Geometry check sheet. Reference: the model listing, model coordinates, mm. A direction names the side the tool comes from. Give positions to 0.01 mm unless a question says otherwise; leave off trailing zeros. Loops run counter-clockwise (first coordinate to the right, second up) from the corner with the lowest first, then second, coordinate; pieces in that order, holes last.
1. Cross-section at A-A, the plane y = 12.5. Record the cut outline in (x, z).
2. Cross-section at B-B, the plane z = -22.25. Record the cut outline in (x, y).
3. Release check for a two-part mould opening along X. For faces 1 (the flat face through (-29.572, 12.3, -31.3)), 2 (the flat face through (-14.5, 25, -38.8)), 3 (the cylindrical face through (-2.767, 22.487, -38.843)) record: +X half, -X half, draft (parallel to the pull), parting line (faces both ways), or undercut.
4. Tool access check on faces 4 (the cylindrical face through (-21.14, 4.45, -38.84)), 5 (the flat face through (-29.072, 12.3, -31.3)). Record the directions out of +Z, -Z, +X, -X, +Y, -Y that give a thin tool (end or side, any length) a straight path to the whole face; none if there is none.
5. Cross-section at D-D, the plane x = -2.5. Record the cut outline in (y, z).
6. Material ranges on L1, parallel to Z at x = -22.5, y = 1.5; L2, parallel to X at y = 24, z = -26.25, recorded low to high.
7. Cross-section at C-C, the plane y = 4. Record the cut outline in (x, z), plus the area to 3 significant figures.
8. Go/stop test with flat-tipped pins: pin 1 Ø7.5 at (x, y) = (-10, 14) entering from +Z; pin 2 Ø12.5 at (y, z) = (10.5, -24) entering from +X. Record where each tip stops, or that it passes through.
Autodesk Inventor part; units mm, degrees
ref_plane "YZ Plane" through (0, 0, 0) normal (1, 0, 0) x (0, 1, 0)
ref_plane "XZ Plane" through (0, 0, 0) normal (0, 1, 0) x (-1, 0, 0)
ref_plane "XY Plane" through (0, 0, 0) normal (0, 0, 1) x (1, 0, 0)
sketch "草圖1" plane through (0, 0, 0) normal (0, 1, 0) x (-1, 0, 0)
  line L0 (29.5719, -39.0966) -> (29.5719, -13.0966)
  line L1 (29.5719, -39.0966) -> (-0.4281, -39.0966)
  point P0 (0, 0)
  dimension "d0" = 26
  dimension "d2" = 90
  dimension "d3" = 30
contour flange "輪廓線凸緣1" sketch "草圖1" thickness 0.5 bend radius 0.5 width 25 along (0, 1, 0) mid plane no both sides no wall seen from (-29.5719, 0, -26.0966) lies toward (1, 0, 0) curves L0 L1
bend "折彎1"
corner "轉角1"
sketch "草圖2" plane through (-29.0719, 0, -13.0966) normal (1, 0, 0) x (0, 0, -1)
  circle A0 centre (12.5, 12.5) radius 12.5
  line L0 (0, 25) -> (25, 25)
  line L1 (0, 0) -> (0, 25)
  line L2 (0, 0) -> (25, 0)
  point P0 (-13.0966, 0)
  point P1 (0, 12.5)
  point P2 (12.5, 25)
  point P3 (12.5, 0)
  dimension "d15" = 25
extrude "擠出1" cut sketch "草圖2" against normal up to surface (0.5 mm away) contours A0 L1 L0 | L2 L1 A0
sketch "草圖3" plane through (-29.0719, 0, -38.0966) normal (1, 0, 0) x (0, 0, -1)
  arc A0 (-12.5, 25) -> (-12.5, 0) centre (-12.5, 12.5) ccw
  circle A1 centre (-12.5, 21) radius 1.5
  circle A2 centre (-12.5, 4) radius 1.5
  point P0 (-38.0966, 0)
  dimension "d18" = 3
  dimension "d19" = 17
  dimension "d20" = 8.5
  dimension "d21" = 3
extrude "擠出2" cut sketch "草圖3" against normal up to surface (0.5 mm away)
sketch "草圖4" plane through (0.4281, 0, -38.5966) normal (0, 0, 1) x (1, 0, 0)
  circle A0 centre (-23, 21) radius 1.5
  circle A1 centre (-3, 21) radius 1.5
  circle A2 centre (-23, 4) radius 1.5
  circle A3 centre (-3, 4) radius 1.5
  line L0 (0, 0) -> (0, 25)
  line L1 (-3, 21) -> (-3, 4)
  line L2 (-3, 12.5) -> (-13.1347, 12.5)
  line L3 (-29, 25) -> (0, 25)
  point P0 (-0.4281, 0)
  dimension "d24" = 20
  dimension "d25" = 3
  dimension "d26" = 3
  dimension "d27" = 3
  dimension "d28" = 3
  dimension "d29" = 17
  dimension "d30" = 3
  dimension "d31" = 12.5
extrude "擠出3" cut sketch "草圖4" against normal up to surface (0.5 mm away)
sketch "草圖5" plane through (-29.0719, 0, -38.0966) normal (1, 0, 0) x (0, 0, -1)
  arc A0 (-12.5, 25) -> (-12.5, 0) centre (-12.5, 12.5) ccw
  circle A1 centre (-12.5, 12.5) radius 5.5
  point P0 (-38.0966, 0)
  dimension "d34" = 11
extrude "擠出4" cut sketch "草圖5" against normal up to surface (0.5 mm away)
equation "\"d4\" = 厚度"
equation "\"d5\" = 折彎離隙寬度"
equation "\"d6\" = 折彎離隙深度"
equation "\"d7\" = 最小剩餘"
equation "\"d8\" = 轉移半徑"
equation "\"d10\" = 折彎半徑"
equation "\"d12\" = 轉角離隙大小"
equation "\"d13\" = 間隙大小"
equation "\"d14\" = Jacobi半徑大小"
equation "\"折彎半徑\" = 厚度"
equation "\"折彎離隙寬度\" = 厚度"
equation "\"折彎離隙深度\" = 0.5 * 厚度"
equation "\"轉角離隙大小\" = 4 * 厚度"
equation "\"最小剩餘\" = 2 * 厚度"
equation "\"轉移半徑\" = 折彎半徑"
equation "\"Jacobi半徑大小\" = 折彎半徑"
equation "\"間隙大小\" = 厚度"
properties part number "wheel_base"
Result:
1. outline: (-29.57, -38.1) arc R1 ccw to (-28.57, -39.1) - (0.43, -39.1) - (0.43, -38.6) - (-28.57, -38.6) arc R0.5 cw to (-29.07, -38.1) - (-29.07, -31.1) - (-29.57, -31.1) - close; (-29.57, -20.1) - (-29.07, -20.1) - (-29.07, -13.1) - (-29.57, -13.1) - close
2. outline: (-29.57, 0.46) - (-29.07, 0.46) - (-29.07, 8.14) - (-29.57, 8.14) - close; (-29.57, 16.86) - (-29.07, 16.86) - (-29.07, 24.54) - (-29.57, 24.54) - close
3. face 1: -X half
3. face 2: draft
3. face 3: undercut
4. face 4: +Z, -Z
4. face 5: +Z, +X, +Y, -Y
5. outline: (0, -39.1) - (2.5, -39.1) - (2.5, -38.6) - (0, -38.6) - close; (5.5, -39.1) - (19.5, -39.1) - (19.5, -38.6) - (5.5, -38.6) - close; (22.5, -39.1) - (25, -39.1) - (25, -38.6) - (22.5, -38.6) - close
6. L1: z = -39.1 to -38.6
6. L2: x = -29.57 to -29.07
7. outline: (-29.57, -38.1) arc R1 ccw to (-28.57, -39.1) - (-24.07, -39.1) - (-24.07, -38.6) - (-28.57, -38.6) arc R0.5 cw to (-29.07, -38.1) - (-29.07, -27.1) - (-29.57, -27.1) - close; (-29.57, -24.1) - (-29.07, -24.1) - (-29.07, -16.43) - (-29.57, -16.43) - close; (-21.07, -39.1) - (-4.07, -39.1) - (-4.07, -38.6) - (-21.07, -38.6) - close; (-1.07, -39.1) - (0.43, -39.1) - (0.43, -38.6) - (-1.07, -38.6) - close
7. area: 21.4 mm2
8. pin 1: stops at z = -38.6
8. pin 2: stops at x = -29.07
